Geometry check sheet. Reference: the model listing, model coordinates, mm. A direction names the side the tool comes from. Give positions to 0.01 mm unless a question says otherwise; leave off trailing zeros. Order: outer loops, then holes, each group sorted by start corner. A loop starts at its lowest first (then second) coordinate and runs counter-clockwise, first axis right, second up. Notation, with made-up numbers: M -29,-29.5 L 12,-29.5 A17 ccw 12,-3.5 Z; hole C 69.25,78.5 d6. An arc over 180 degrees is marked long. Answer as CSV lines item,"result". Start each with the question number.
Q1. Thickness scan on line 1 (Y direction, x = 3.5, z = 3.75); line 2 (Y direction, x = 9, z = -6.75); line 3 (Y direction, x = 17.5, z = 8). Record the ranges inside material, lowest first.
Q2. Section check D-D, the plane y = 4. Record the boundary of the cut face in (x, z) (3 decimals), then the cut area to 3 significant figures.
Q3. Mould release check, pull along X, two halves, no side actions. Record for faces 1 (the flat face through (12, 0, -12.6)), 2 (the flat face through (3, 0, 13.75)), 3 (the cylindrical face through (0.285, 19.699, -0.193)), 4 (the flat face through (4.68, 0, 13)): +X half, -X half, draft (parallel to the pull), parting line (faces both ways), or undercut.
Q4. Section check C-C, the plane z = -3.5. Record the boundary of the cut face in (x, y), then the cut area to 3 significant figures.
Q5. Section check A-A, the plane y = 15. Record the boundary of the cut face in (x, z).
Q6. Set-up check for faces 5 (the flat face through (15, 9, 0)), 6 (the flat face through (3, 0, 12.425)), 7 (the flat face through (12, -5.325, 13)), 8 (the flat face through (5, 11.9, 0)): record each of +Z, -Z, +X, -X, +Y, -Y from which the full face is reachable in a straight line by a thin tool's end or side.
Q7. Go/stop test with flat-tipped pins: pin 1 (0.9 mm diameter, centred on x = 17, z = -13, fed in from -Y); pin 2 (0.6 mm diameter, centred on y = 0.5, z = -13.5, fed in from +X); pin 3 (4 mm diameter, centred on y = -0.5, z = -2.5, fed in from -X). Record where each tip stops, or that it passes through.
Q8. Section check B-B, the plane x = 7.5. Record the boundary of the cut face in (y, z) (3 decimals), then the cut area to 3 significant figures.
Autodesk Inventor part; units mm, degrees
ref_plane "side_1_XY" through (0, 0, 0) normal (-1, 0, 0) x (0, 0, -1)
ref_plane "side_1_YZ" through (0, 0, 0) normal (0, 0, -1) x (0, -1, 0)
ref_plane "side_1_ZX" through (0, 0, 0) normal (0, -1, 0) x (-1, 0, 0)
sketch "Skizze_1" plane through (0, 0, 0) normal (0, 0, 1) x (1, 0, 0)
  line L0 (0, 19) -> (0, -19)
  arc A0 (0, -19) -> (1, -20) centre (1, -19) ccw
  line L1 (1, -20) -> (9, -20)
  arc A1 (9, -20) -> (10, -19) centre (9, -19) ccw
  line L2 (10, -19) -> (10, -10)
  arc A2 (11, -9) -> (10, -10) centre (11, -10) ccw
  line L3 (11, -9) -> (19, -9)
  arc A3 (19, -9) -> (20, -8) centre (19, -8) ccw
  line L4 (20, -8) -> (20, 8)
  arc A4 (20, 8) -> (19, 9) centre (19, 8) ccw
  line L5 (19, 9) -> (11, 9)
  arc A5 (10, 10) -> (11, 9) centre (11, 10) ccw
  line L6 (10, 10) -> (10, 19)
  arc A6 (10, 19) -> (9, 20) centre (9, 19) ccw
  line L7 (9, 20) -> (1, 20)
  arc A7 (1, 20) -> (0, 19) centre (1, 19) ccw
extrude "Extrusion1" add sketch "Skizze_1" along normal mid plane 27.5
sketch "Skizze_2" plane through (0, 0, 0) normal (1, 0, 0) x (0, 1, 0)
  arc A0 (18.1, 6.5) -> (11.9, 6.5) centre (15, 6.5) ccw
  line L0 (11.9, 6.5) -> (11.9, -6.5)
  arc A1 (11.9, -6.5) -> (18.1, -6.5) centre (15, -6.5) ccw
  line L1 (18.1, -6.5) -> (18.1, 6.5)
extrude "Extrusion2" cut sketch "Skizze_2" along normal blind 10
sketch "Skizze_3" plane through (0, 0, 0) normal (1, 0, 0) x (0, 1, 0)
  arc A0 (-11.9, 6.5) -> (-18.1, 6.5) centre (-15, 6.5) ccw
  line L0 (-18.1, 6.5) -> (-18.1, -6.5)
  arc A1 (-18.1, -6.5) -> (-11.9, -6.5) centre (-15, -6.5) ccw
  line L1 (-11.9, -6.5) -> (-11.9, 6.5)
extrude "Extrusion3" cut sketch "Skizze_3" along normal blind 10
sketch "Skizze_4" plane through (20, 0, 0) normal (1, 0, 0) x (0, 0, -1)
  line L0 (-13.75, 5.325) -> (-13.75, -5.325)
  line L1 (-13.75, -5.325) -> (-12.6, -5.325)
  line L2 (-12.6, -5.325) -> (-12.6, 5.325)
  line L3 (-12.6, 5.325) -> (-13.75, 5.325)
extrude "Extrusion4" cut sketch "Skizze_4" against normal blind 15.32
sketch "Skizze_5" plane through (20, 0, 0) normal (1, 0, 0) x (0, 0, -1)
  line L0 (12.6, 3.4) -> (12.6, -3.4)
  line L1 (12.6, -3.4) -> (13.75, -3.4)
  line L2 (13.75, -3.4) -> (13.75, 3.4)
  line L3 (13.75, 3.4) -> (12.6, 3.4)
extrude "Extrusion5" cut sketch "Skizze_5" against normal blind 15.32
sketch "Skizze_6" plane through (0, 0, 0) normal (0, 1, 0) x (-1, 0, 0)
  line L0 (-6.5, 8.75) -> (-6.5, 13.75)
  line L1 (-6.5, 13.75) -> (-8.5, 13.75)
  line L2 (-8.5, 13.75) -> (-8.5, 11.75)
  line L3 (-8.5, 11.75) -> (-15.5, 11.75)
  line L4 (-15.5, 11.75) -> (-15.5, 13.75)
  line L5 (-15.5, 13.75) -> (-17.5, 13.75)
  line L6 (-17.5, 13.75) -> (-17.5, 8.75)
  line L7 (-17.5, 8.75) -> (-6.5, 8.75)
extrude "Extrusion6" add sketch "Skizze_6" along normal mid plane 10
sketch "Skizze_7" plane through (0, 0, 0) normal (0, 1, 0) x (-1, 0, 0)
  line L0 (-6.5, -8.75) -> (-17.5, -8.75)
  line L1 (-17.5, -8.75) -> (-17.5, -13.75)
  line L2 (-17.5, -13.75) -> (-15.5, -13.75)
  line L3 (-15.5, -13.75) -> (-15.5, -11.75)
  line L4 (-15.5, -11.75) -> (-8.5, -11.75)
  line L5 (-8.5, -11.75) -> (-8.5, -13.75)
  line L6 (-8.5, -13.75) -> (-6.5, -13.75)
  line L7 (-6.5, -13.75) -> (-6.5, -8.75)
extrude "Extrusion7" add sketch "Skizze_7" along normal mid plane 6.75
sketch "Skizze_8" plane through (0, 0, 0) normal (1, 0, 0) x (0, 1, 0)
  line L0 (7.5, 12.425) -> (-7.5, 12.425)
  line L1 (-7.5, 12.425) -> (-7.5, -12.425)
  line L2 (-7.5, -12.425) -> (7.5, -12.425)
  line L3 (7.5, -12.425) -> (7.5, 12.425)
extrude "Extrusion8" cut sketch "Skizze_8" along normal blind 6
ref_plane "side_1_XY" through (0, 0, 0) normal (-1, 0, 0) x (0, 0, -1)
ref_plane "side_1_YZ" through (0, 0, 0) normal (0, 0, -1) x (0, -1, 0)
ref_plane "side_1_ZX" through (0, 0, 0) normal (0, -1, 0) x (-1, 0, 0)
properties part number "May Tec 1.65.2101_Magnetic lock PA 0"
Answer block:
1,line 1,"y = -20 to -18.1, -11.9 to -7.5, 7.5 to 11.9, 18.1 to 20"
1,line 2,"y = -20 to -18.09, -11.91 to 11.91, 18.09 to 20"
1,line 3,"y = -9 to 9"
2,outline,"M 0,-13.75 L 20,-13.75 L 20,12.6 L 17.5,12.6 L 17.5,13.75 L 15.5,13.75 L 15.5,12.6 L 8.5,12.6 L 8.5,13.75 L 6.5,13.75 L 6.5,12.6 L 4.68,12.6 L 4.68,13.75 L 0,13.75 L 0,12.425 L 6,12.425 L 6,-12.425 L 0,-12.425 Z"
2,area,"388 mm2"
3,face 1,"undercut"
3,face 2,"draft"
3,face 3,"-X half"
3,face 4,"undercut"
4,outline,"M 0,-19 A1 ccw 1,-20 L 9,-20 A1 ccw 10,-19 L 10,-18.1 L 0,-18.1 Z; M 0,-11.9 L 10,-11.9 L 10,-10 A1 cw 11,-9 L 19,-9 A1 ccw 20,-8 L 20,8 A1 ccw 19,9 L 11,9 A1 cw 10,10 L 10,11.9 L 0,11.9 L 0,7.5 L 6,7.5 L 6,-7.5 L 0,-7.5 Z; M 0,18.1 L 10,18.1 L 10,19 A1 ccw 9,20 L 1,20 A1 ccw 0,19 Z"
4,area,"365 mm2"
5,outline,"M 0,-13.75 L 10,-13.75 L 10,-9.6 L 0,-9.6 Z; M 0,9.6 L 10,9.6 L 10,13.75 L 0,13.75 Z"
6,face 5,"+Z, -Z, +X, +Y"
6,face 6,"-X"
6,face 7,"+Z, +X"
6,face 8,"+X, -X"
7,pin 1,"stops at y = -9"
7,pin 2,"stops at x = 17.5"
7,pin 3,"stops at x = 6"
8,outline,"M -20,-13.75 L -3.4,-13.75 L -3.4,-12.6 L -3.375,-12.6 L -3.375,-13.75 L 3.375,-13.75 L 3.375,-12.6 L 3.4,-12.6 L 3.4,-13.75 L 20,-13.75 L 20,13.75 L 5.325,13.75 L 5.325,12.6 L 5,12.6 L 5,13.75 L -5,13.75 L -5,12.6 L -5.325,12.6 L -5.325,13.75 L -20,13.75 Z; hole M -18.1,-6.5 A3.1 ccw -11.9,-6.5 L -11.9,6.5 A3.1 ccw -18.1,6.5 Z; hole M 11.9,-6.5 A3.1 ccw 18.1,-6.5 L 18.1,6.5 A3.1 ccw 11.9,6.5 Z"
8,area,"878 mm2"
